For this review, take the finished solid that the model builds, in its own axes (mm). A direction names the side the tool comes from. Give positions to 0.01 mm unless a question says otherwise; leave off trailing zeros. Loops run counter-clockwise (first coordinate to the right, second up) from the corner with the lowest first, then second, coordinate; pieces in that order, holes last.
```python
from build123d import *
from build123d import SkipClean  # not in build123d's __all__

# Parameters (mm, degrees)
F1_DEPTH  = 40
F2_DEPTH  = 3
F3_DEPTH  = 24
F4_DEPTH  = 40
F6_DEPTH  = 2.5
F7_W      = 6
F7_H      = 1.3
F8_DEPTH  = 13
F9_W      = 4
F9_H      = 2
F10_DEPTH = 6.5
F11_R     = 1.5
F12_DEPTH = 3.5
F13_R     = 5
F14_DEPTH = 2.5
F15_R     = 3.8627416998
F16_R     = 7
F17_R     = 7
F18_R     = 5


# Not quite as in the source:
# - after a boolean that leaves OpenCascade's solid faulty, fix() repairs it


with BuildPart() as f1:
    # F0 (on Top) → F1 (new body)
    with BuildSketch(Plane.XY):
        with BuildLine():
            ThreePointArc((136.0017471959, 19.0444356012), (93.4644134414, 27.0237675476), (58.1274125485, 52.0115819608))
            ThreePointArc((58.1274125485, 52.0115819608), (-1.3417961939, 78.0013424722), (-59.8907435455, 49.9999995776))
            ThreePointArc((-59.8907435455, 49.9999995776), (-77.9889397002, -0.003066533), (-59.8738076097, -49.9999995776))
            ThreePointArc((-59.8738076097, -49.9999995776), (-1.3426138919, -77.9810495035), (58.1087045089, -52.0122117666))
            ThreePointArc((58.1087045089, -52.0122117666), (93.4442134492, -27.0247840784), (135.9799137778, -19.0445627716))
            Line((135.9799137778, -19.0445627716), (136.0017471959, 19.0444356012))
        make_face()
        with BuildLine():
            ThreePointArc((55.9016994375, 50), (90.8688121766, 24.8773821457), (133, 16))
            Line((133, 16), (132.9816567922, -16.0002304621))
            ThreePointArc((132.9816567922, -16.0002304621), (90.8504689689, -24.8776126078), (55.8833562297, -50.0002304621))
            ThreePointArc((55.8833562297, -50.0002304621), (-75.0149890076, 0.0238973514), (55.9016994375, 50))
        make_face(mode=Mode.SUBTRACT)
    extrude(amount=F1_DEPTH)

    # F0 (on Top) → F2 (join)
    with BuildSketch(Plane.XY):
        with BuildLine():
            ThreePointArc((136.0017471959, 19.0444356012), (93.4644134414, 27.0237675476), (58.1274125485, 52.0115819608))
            ThreePointArc((58.1274125485, 52.0115819608), (-1.3417961939, 78.0013424722), (-59.8907435455, 49.9999995776))
            ThreePointArc((-59.8907435455, 49.9999995776), (-77.9889397002, -0.003066533), (-59.8738076097, -49.9999995776))
            ThreePointArc((-59.8738076097, -49.9999995776), (-1.3426138919, -77.9810495035), (58.1087045089, -52.0122117666))
            ThreePointArc((58.1087045089, -52.0122117666), (93.4442134492, -27.0247840784), (135.9799137778, -19.0445627716))
            Line((135.9799137778, -19.0445627716), (136.0017471959, 19.0444356012))
        make_face()
        with BuildLine():
            ThreePointArc((55.9016994375, 50), (90.8688121766, 24.8773821457), (133, 16))
            Line((133, 16), (132.9816567922, -16.0002304621))
            ThreePointArc((132.9816567922, -16.0002304621), (90.8504689689, -24.8776126078), (55.8833562297, -50.0002304621))
            ThreePointArc((55.8833562297, -50.0002304621), (-75.0149890076, 0.0238973514), (55.9016994375, 50))
        make_face(mode=Mode.SUBTRACT)
        with BuildLine():
            ThreePointArc((-59.8738076097, -49.9999995776), (-77.9889397002, -0.003066533), (-59.8907435455, 49.9999995776))
            ThreePointArc((-59.8907435455, 49.9999995776), (-78.014990719, -0.003070945), (-59.8738076097, -49.9999995776))
        make_face()
        with BuildLine():
            Line((106.9816567922, 16), (133, 16))
            ThreePointArc((133, 16), (90.8688121766, 24.8773821457), (55.9016994375, 50))
            ThreePointArc((55.9016994375, 50), (-75.0149890076, 0.0238973514), (55.8833562297, -50.0002304621))
            ThreePointArc((55.8833562297, -50.0002304621), (90.8504689689, -24.8776126078), (132.9816567922, -16.0002304621))
            Line((132.9816567922, -16.0002304621), (106.9816567922, -16.0002304621))
            Line((106.9816567922, -16.0002304621), (106.9816567922, 16))
        make_face()
        Polygon((71.8, 25.4997695379), (85.881656831, 25.4997695379), (85.881656831, 15.3997695379), (78.2822565953, 15.3042914831), (78.2659248228, 16.6041888918), (84.6000000387, 16.6837695379), (84.6000000387, 24.1997695379), (73.1, 24.1997695379), (73.1, -24.2002304621), (84.6000000387, -24.2002304621), (84.6000000387, -16.6047524073), (78.2822565953, -16.6047524073), (78.2822565953, -15.3047524073), (85.881656831, -15.4002304621), (85.881656831, -25.5002304621), (71.8, -25.5002304621), align=None, mode=Mode.SUBTRACT)
        Polygon((132.9816567922, -16.0002304621), (133, 16), (106.9816567922, 16), (106.9816567922, -16.0002304621), align=None)
        Polygon((109.1000003293, -13.881886925), (109.1000003293, 13.8816564629), (130.8804418356, 13.8816564629), (130.8645271863, -13.881886925), align=None, mode=Mode.SUBTRACT)
        Polygon((130.8804418356, 13.8816564629), (109.1000003293, 13.8816564629), (109.1000003293, -13.881886925), (130.8645271863, -13.881886925), align=None)
        Polygon((85.881656831, 15.3997695379), (85.881656831, 25.4997695379), (71.8, 25.4997695379), (71.8, -25.5002304621), (85.881656831, -25.5002304621), (85.881656831, -15.4002304621), (78.2822565953, -15.3047524073), (78.2822565953, -16.6047524073), (84.6000000387, -16.6047524073), (84.6000000387, -24.2002304621), (73.1, -24.2002304621), (73.1, 24.1997695379), (84.6000000387, 24.1997695379), (84.6000000387, 16.6837695379), (78.2659248228, 16.6041888918), (78.2822565953, 15.3042914831), align=None)
    with SkipClean():  # cleaning this boolean's faces spoils the solid; the shape is the same uncleaned
        extrude(amount=-F2_DEPTH)

    # F0 (on Top) → F3 (join)
    with BuildSketch(Plane.XY):
        Polygon((85.881656831, 15.3997695379), (85.881656831, 25.4997695379), (71.8, 25.4997695379), (71.8, -25.5002304621), (85.881656831, -25.5002304621), (85.881656831, -15.4002304621), (78.2822565953, -15.3047524073), (78.2822565953, -16.6047524073), (84.6000000387, -16.6047524073), (84.6000000387, -24.2002304621), (73.1, -24.2002304621), (73.1, 24.1997695379), (84.6000000387, 24.1997695379), (84.6000000387, 16.6837695379), (78.2659248228, 16.6041888918), (78.2822565953, 15.3042914831), align=None)
    extrude(amount=F3_DEPTH)

    add(f1.part.fix(), mode=Mode.REPLACE)

    # F0 (on Top) → F4 (join)
    with BuildSketch(Plane.XY):
        Polygon((132.9816567922, -16.0002304621), (133, 16), (106.9816567922, 16), (106.9816567922, -16.0002304621), align=None)
        Polygon((109.1000003293, -13.881886925), (109.1000003293, 13.8816564629), (130.8804418356, 13.8816564629), (130.8645271863, -13.881886925), align=None, mode=Mode.SUBTRACT)
    extrude(amount=F4_DEPTH)

    # F5 (on face) → F6 (cut)
    with BuildSketch(Plane(origin=(71.8, 0, 0), x_dir=(0, -1, 0), z_dir=(-1, 0, 0))):
        with BuildLine():
            Line((19.7002304621, 24), (-19.6997695379, 24))
            ThreePointArc((-19.6997695379, 24), (0.0002304621, 3.4999999987), (19.7002304621, 24))
        make_face()
    extrude(amount=-F6_DEPTH, mode=Mode.SUBTRACT)

    # F7 (on face) → F8 (join)
    with BuildSketch(Plane.XY):
        with Locations((97.1279456019, 6.8092534184)):
            Rectangle(F7_W, F7_H)
        with Locations((97.1279456019, -6.85)):
            Rectangle(F7_W, F7_H)
    extrude(amount=F8_DEPTH)

    # F9 (on face) → F10 (join)
    with BuildSketch(Plane.XY):
        with Locations((78.6196921468, 9)):
            Rectangle(F9_W, F9_H)
        with Locations((78.6196921468, -9)):
            Rectangle(F9_W, F9_H)
    extrude(amount=F10_DEPTH)

    # F11 (on face) → F12 (cut)
    with BuildSketch(Plane(origin=(106.9816567922, 0, 0), x_dir=(0, -1, 0), z_dir=(-1, 0, 0))):
        with Locations((0.0001152311, 28)):
            Circle(F11_R)
    extrude(amount=-F12_DEPTH, mode=Mode.SUBTRACT)

    # F13 (on face) → F14 (cut)
    with BuildSketch(Plane(origin=(106.9816567922, 0, 0), x_dir=(0, -1, 0), z_dir=(-1, 0, 0))):
        with Locations((0, 11.5517321974)):
            Circle(F13_R)
    extrude(amount=-F14_DEPTH, mode=Mode.SUBTRACT)

    # F15
    f15_edges = [f1.edges().sort_by_distance(p)[0] for p in [
        (130.880442, 13.881656, 20),
        (106.981657, 16, 20),
        (109.1, 13.881656, 20),
        (130.864527, -13.881887, 20),
        (106.981657, -16.00023, 20),
        (109.1, -13.881887, 20),
    ]]
    fillet(f15_edges, radius=F15_R)

    # F16
    f16_edges = [f1.edges().sort_by_distance(p)[0] for p in [
        (132.981657, -16.00023, 20),
    ]]
    fillet(f16_edges, radius=F16_R)

    # F17
    f17_edges = [f1.edges().sort_by_distance(p)[0] for p in [
        (133, 16, 20),
    ]]
    fillet(f17_edges, radius=F17_R)

    # F18
    f18_edges = [f1.edges().sort_by_distance(p)[0] for p in [
        (135.979914, -19.044563, 18.5),
        (136.001747, 19.044436, 18.5),
    ]]
    fillet(f18_edges, radius=F18_R)


solid = f1.part
```
Q1. For pin 1 Ø5 at (x, z) = (96, 3.5) entering from +Y; pin 2 Ø0.7 at (y, z) = (-15.5, 15) entering from -X; pin 3 Ø4 at (x, z) = (79, 19.5) entering from +Y, all flat-tipped, find the tip position at first contact; note any pin that passes through.
Answers:
pin 1: stops at y = 27.01
pin 2: stops at x = -76.5
pin 3: stops at y = 35.86
Q2. Mouldability with a two-part tool opening along Y and no side actions: class faces 4 (the flat face through (68, 41, 40)), 5 (the cylindrical face through (134.512, -17.561, 18.199)), 6 (the cylindrical face through (-74.973, -2.508, 19.72)) as +Y half, -Y half, draft (parallel to the pull), parting line (faces both ways), or undercut.
Answers:
face 4: draft
face 5: -Y half
face 6: undercut
Q3. Consider section D-D on y = 61.5. Give the boundary of the cut face in (x, z), plus the area to 3 significant figures.
Answers:
outline: (-48.01, -3) - (47.98, -3) - (47.98, 40) - (42.93, 40) - (42.93, 0) - (-42.96, 0) - (-42.96, 40) - (-48.01, 40) - close
area: 692 mm2
Q4. For probe 1 along X at (y, z) = (2, 25); probe 2 along Z at (x, y) = (108, 0); probe 3 along Y at (x, z) = (-1, 21.5), list the stretches that pass through material, from the lowest coordinate up.
Answers:
probe 1: x = -77.96 to -74.99, 106.98 to 109.1, 130.87 to 135.99
probe 2: z = -3 to 6.55, 16.55 to 26.5, 29.5 to 40
probe 3: y = -77.99 to -74.99, 75.01 to 78.01
Q5. Consider section C-C on z = 19.5. Count the separate pieces of the cut face and the enclosed holes in it, plus the area to 3 significant figures.
Answers:
separate pieces: 3
enclosed holes: 2
area: 2,120 mm2
Q6. Consider section B-B on x = 40. Give the boundary of the cut face in (y, z).
Answers:
outline: (-66.95, -3) - (66.97, -3) - (66.97, 40) - (63.45, 40) - (63.45, 0) - (-63.43, 0) - (-63.43, 40) - (-66.95, 40) - close
Q7. Machinability: for faces 1 (the cylindrical face through (91.741, 27.772, 18.801)), 2 (the cylindrical face through (108.03, 0.65, 16.51)), 3 (the flat face through (84.6, 20, 12)), which of the approach directions +Z, -Z, +X, -X, +Y, -Y give a long, thin tool a straight path to every point of the face, cutting with its end or side? Answer none if there is none.
Answers:
face 1: +Z, -Z, +X, +Y
face 2: none
face 3: +Z
